```python
from build123d import *

# Parameters (mm, degrees)
BOSS_EXTRUDE1_DEPTH = 1000
SKETCH2_W           = 45
SKETCH2_H           = 130
BOSS_EXTRUDE2_DEPTH = 145
CHAMFER1_SIZE       = 3


with BuildPart() as part:
    # Sketch1 → Boss-Extrude1 (new body)
    with BuildSketch(Plane.XY):
        Polygon((-8.548454956, 0), (-50, 0), (-50, -40), (150, -40), (150, 0), (131.451545044, 0), (100, 0), (100, -10), (120, -10), (120, -20), (65, -20), (65, -10), (80, -10), (80, 0), (77.428634929, 0), (47.428634929, 0), (20, 0), (20, -10), (35, -10), (35, -20), (-20, -20), (-20, -10), (0, -10), (0, 0), align=None)
    extrude(amount=BOSS_EXTRUDE1_DEPTH)

    # Sketch2 → Boss-Extrude2 (add)
    with BuildSketch(Plane.XZ.offset(40)):
        with Locations((127.5, 935)):
            Rectangle(SKETCH2_W, SKETCH2_H)
        with Locations((-27.5, 935)):
            Rectangle(SKETCH2_W, SKETCH2_H)
        with Locations((127.5, 65)):
            Rectangle(SKETCH2_W, SKETCH2_H)
        with Locations((-27.5, 65)):
            Rectangle(SKETCH2_W, SKETCH2_H)
    extrude(amount=BOSS_EXTRUDE2_DEPTH)

    # Chamfer1
    chamfer1_edges = [part.edges().sort_by_distance(p)[0] for p in [
        (150, 0, 500),
        (-50, 0, 500),
    ]]
    chamfer(chamfer1_edges, length=CHAMFER1_SIZE)


solid = part.part
```
For this review, take the finished solid that the model builds, in its own axes (mm). A direction names the side the tool comes from. Round coordinates to 2 decimals unless told otherwise and drop trailing zeros. Write each loop counter-clockwise with the first axis right and the second up, starting at its lowest first coordinate (ties: lowest second). Pieces come first, ordered by that corner, then holes. Notation, with made-up numbers: (-27, -1.5) -> (4, -1.5) arc R15 ccw to (4, 23.5) -> close; hole circle Ø11 at (17, 65.5). An arc over 180 degrees is marked (long way). Use one line per item in the form item = value.
1) Mouldability with a two-part tool opening along Y and no side actions: class faces 1 (the flat face through (-5, -111, 64)), 2 (the flat face through (127, -185, 936)), 3 (the flat face through (8, -20, 493)), 4 (the flat face through (93, -20, 493)) as +Y half, -Y half, draft (parallel to the pull), parting line (faces both ways), or undercut.
Found:
face_1 = draft
face_2 = -Y half
face_3 = undercut
face_4 = undercut
2) Take a section at A-A, the plane y = -126. Write out the cut boundary in (x, z).
Found:
outline = (-50, 0) -> (-5, 0) -> (-5, 130) -> (-50, 130) -> close; (-50, 870) -> (-5, 870) -> (-5, 1000) -> (-50, 1000) -> close; (105, 0) -> (150, 0) -> (150, 130) -> (105, 130) -> close; (105, 870) -> (150, 870) -> (150, 1000) -> (105, 1000) -> close
3) To check wall thickness, follow L1, parallel to Y at x = 70.5, z = 148; L2, parallel to Z at x = -15, y = -130; L3, parallel to X at y = -68, z = 69. State the ranges of each line that lie inside material, in increasing order. Write a range as from..to.
Found:
L1 = -40..-20, -10..0
L2 = 0..130, 870..1000
L3 = -50..-5, 105..150
4) Tool access review of faces 5 (the flat face through (110, -10, 493)), 6 (the flat face through (127, -111, 130)), 7 (the flat face through (-5, -111, 934)), 8 (the flat face through (127, -185, 66)): name each direction out of +Z, -Z, +X, -X, +Y, -Y from which nothing blocks a thin tool from reaching the whole face with its end or side.
Found:
face_5 = +Z, -Z
face_6 = +X, -X, -Y
face_7 = +Z, -Z, -Y
face_8 = +Z, -Z, +X, -X, -Y
5) Clearance check with flat-ended pins moving along their axes: pin 1 (5 mm diameter, centred on x = 34.5, z = 538, fed in from +Y); pin 2 (22 mm diameter, centred on x = -7.5, z = 611, fed in from -Y). State where each tip first meets the part, or that it passes through.
Found:
pin_1 = 0
pin_2 = -40
6) Take a section at B-B, the plane z = 465.5. Write out the cut boundary in (x, y), and give its area (3 significant figures).
Found:
outline = (-50, -40) -> (150, -40) -> (150, -3) -> (147, 0) -> (100, 0) -> (100, -10) -> (120, -10) -> (120, -20) -> (65, -20) -> (65, -10) -> (80, -10) -> (80, 0) -> (20, 0) -> (20, -10) -> (35, -10) -> (35, -20) -> (-20, -20) -> (-20, -10) -> (0, -10) -> (0, 0) -> (-47, 0) -> (-50, -3) -> close
area = 6,490 mm2
